Geometry check sheet. Reference: drawing and pictorial views, mm from the part's lowest x, y, z. Coordinates: 2 decimals unless noted, no trailing zeros. Order: outer loops, then holes, each group sorted by start corner. A loop starts at its lowest first (then second) coordinate and runs counter-clockwise, first axis right, second up. Notation, with made-up numbers: M 1.5,72.5 L 11.5,72.5 A18 cw 11.5,85.5 Z; hole C 78.5,23.5 d4. An arc over 180 degrees is marked long. Return JSON: item names as keys, results as strings.
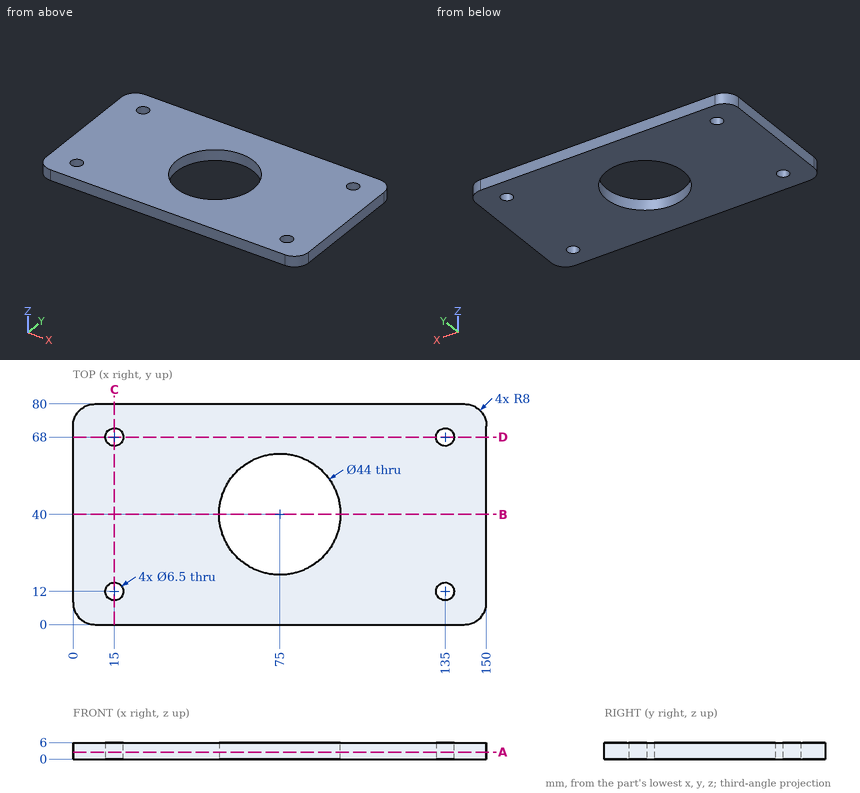
Q1. Cross-section at C-C, the plane x = 15. Record the boundary of the cut face in (y, z).
Values:
{"outline": "M 0,0 L 8.75,0 L 8.75,6 L 0,6 Z; M 15.25,0 L 64.75,0 L 64.75,6 L 15.25,6 Z; M 71.25,0 L 80,0 L 80,6 L 71.25,6 Z"}
Q2. Cross-section at B-B, the plane y = 40. Record the boundary of the cut face in (x, z).
Values:
{"outline": "M 0,0 L 53,0 L 53,6 L 0,6 Z; M 97,0 L 150,0 L 150,6 L 97,6 Z"}
Q3. Cross-section at A-A, the plane z = 2.55. Record the boundary of the cut face in (x, y), and give its area (3 significant figures).
Values:
{"outline": "M 0,8 A8 ccw 8,0 L 142,0 A8 ccw 150,8 L 150,72 A8 ccw 142,80 L 8,80 A8 ccw 0,72 Z; hole C 15,12 d6.5; hole C 15,68 d6.5; hole C 75,40 d44; hole C 135,12 d6.5; hole C 135,68 d6.5", "area": "10,300 mm^2"}
Q4. Material ranges on line 1 along X through (y, z) = (68, 2.6); line 2 along Y through (x, z) = (15, 4.6); line 3 along Y through (x, z) = (134, 2.85), recorded low to high.
Values:
{"line 1": "0 to 11.75, 18.25 to 131.75, 138.25 to 150", "line 2": "0 to 8.75, 15.25 to 64.75, 71.25 to 80", "line 3": "0 to 8.91, 15.09 to 64.91, 71.09 to 80"}
Q5. Cross-section at D-D, the plane y = 68. Record the boundary of the cut face in (x, z), and give its area (3 significant figures).
Values:
{"outline": "M 0,0 L 11.75,0 L 11.75,6 L 0,6 Z; M 18.25,0 L 131.75,0 L 131.75,6 L 18.25,6 Z; M 138.25,0 L 150,0 L 150,6 L 138.25,6 Z", "area": "822 mm^2"}
